Can you work these out from the model? Positions are in its coordinate system, mm. A direction names the side the tool comes from. Round coordinates to 2 decimals unless told otherwise and drop trailing zeros. Loops run counter-clockwise (first coordinate to the right, second up) from the corner with the lowest first, then second, coordinate; pieces in that order, holes last. Notation, with made-up numbers: (74, -2) -> (106, -2) arc R22 ccw to (106, 14) -> close; hole circle Ø7 at (-16.5, 78). An arc over 180 degrees is marked (long way). Answer as a JSON object with one key per item and string values.
```python
from build123d import *

# Parameters (mm, degrees)
SKETCH1_W           = 60
SKETCH1_H           = 45
BOSS_EXTRUDE1_DEPTH = 8
SKETCH2_R           = 5
CUT_EXTRUDE1_DEPTH  = 5
SKETCH3_W           = 20
SKETCH3_H           = 40
CUT_EXTRUDE2_DEPTH  = 5
SKETCH4_W           = 8
SKETCH4_H           = 45
BOSS_EXTRUDE3_DEPTH = 45
SKETCH6_R           = 1.5
CUT_EXTRUDE3_DEPTH  = 45
FILLET2_R           = 2
SKETCH7_R           = 14.99024042
CUT_EXTRUDE4_DEPTH  = 71.10884395


with BuildPart() as part:
    # Sketch1 → Boss-Extrude1 (new body)
    with BuildSketch(Plane(origin=(0, 0, 0), x_dir=(1, 0, 0), z_dir=(0, 1, 0))):
        Rectangle(SKETCH1_W, SKETCH1_H)
    extrude(amount=BOSS_EXTRUDE1_DEPTH)

    # Sketch2 → Cut-Extrude1 (cut)
    with BuildSketch(Plane.XZ):
        with Locations(Location((-20, 14.5, 0), (0, 0, 270))):
            Circle(SKETCH2_R)
        with Locations(Location((-20, -14.5, 0), (0, 0, 270))):
            Circle(SKETCH2_R)
    extrude(amount=-CUT_EXTRUDE1_DEPTH, mode=Mode.SUBTRACT)

    # Sketch3 → Cut-Extrude2 (cut)
    with BuildSketch(Plane.XZ):
        Rectangle(SKETCH3_W, SKETCH3_H)
    extrude(amount=-CUT_EXTRUDE2_DEPTH, mode=Mode.SUBTRACT)

    # Sketch4 → Boss-Extrude3 (add)
    with BuildSketch(Plane(origin=(0, 8, 0), x_dir=(1, 0, 0), z_dir=(0, 1, 0))):
        with Locations((-6, 0)):
            Rectangle(SKETCH4_W, SKETCH4_H)
    extrude(amount=BOSS_EXTRUDE3_DEPTH)

    # Sketch6 → Cut-Extrude3 (cut)
    with BuildSketch(Plane.ZY.offset(10)):
        with Locations((-15, 45.5)):
            Circle(SKETCH6_R)
        with Locations((15, 45.5)):
            Circle(SKETCH6_R)
        with Locations((15, 15.5)):
            Circle(SKETCH6_R)
        with Locations((-15, 15.5)):
            Circle(SKETCH6_R)
    extrude(amount=-CUT_EXTRUDE3_DEPTH, mode=Mode.SUBTRACT)

    # Fillet2
    fillet2_edges = [part.edges().sort_by_distance(p)[0] for p in [
        (-6, 53, -22.5),
        (-6, 53, 22.5),
    ]]
    fillet(fillet2_edges, radius=FILLET2_R)

    # Sketch7 → Cut-Extrude4 (cut, through all)
    with BuildSketch(Plane.ZY.offset(10)):
        with Locations((0, 30.5)):
            Circle(SKETCH7_R)
    extrude(amount=-CUT_EXTRUDE4_DEPTH, mode=Mode.SUBTRACT)


solid = part.part
```
Q1. We'd pull the mould along Z, two halves only. Please class faces 1 (the cylindrical face through (-24.88, 2.46, 15.58)), 2 (the flat face through (-2.4, 14, 22.5)), 3 (the flat face through (-6, 53, 0)): pulls with the +Z half, pulls with the -Z half, needs draft (parallel to the pull), parting line crosses it, or undercut.
Determined:
{"face 1": "undercut", "face 2": "pulls with the +Z half", "face 3": "needs draft"}
Q2. If I drill on L1, parallel to X at y = 2.5, z = 8.5; L2, parallel to X at y = 47, z = -10; L3, parallel to Y at x = -7, z = 0, over which ranges is the centre line in solid material (lowest first)? Write a range as [from, to].
Determined:
{"L1": "[-30, -10], [10, 30]", "L2": "[-10, -2]", "L3": "[5, 15.51], [45.49, 53]"}
Q3. I want a section at D-D, the plane z = 11. Write out the boundary of the cut face in (x, y).
Determined:
{"outline": "(-30, 0) -> (-23.57, 0) -> (-23.57, 5) -> (-16.43, 5) -> (-16.43, 0) -> (-10, 0) -> (-10, 5) -> (10, 5) -> (10, 0) -> (30, 0) -> (30, 8) -> (-2, 8) -> (-2, 20.32) -> (-10, 20.32) -> (-10, 8) -> (-30, 8) -> close; (-10, 40.68) -> (-2, 40.68) -> (-2, 53) -> (-10, 53) -> close"}
Q4. I want a section at C-C, the plane y = 33.5. Write out the boundary of the cut face in (x, z), then the cut area to 3 significant figures.
Determined:
{"outline": "(-10, -22.5) -> (-2, -22.5) -> (-2, -14.69) -> (-10, -14.69) -> close; (-10, 14.69) -> (-2, 14.69) -> (-2, 22.5) -> (-10, 22.5) -> close", "area": "125 mm²"}
Q5. I'm going to push flat-ended pins straight in: pin 1 (4 mm diameter, centred on y = 11.5, z = 7.5, fed in from +X); pin 2 (1.8 mm diameter, centred on y = 15.5, z = -15, fed in from -X); pin 3 (9 mm diameter, centred on x = -20, z = -14.5, fed in from +Y); pin 4 (10 mm diameter, centred on x = 1.5, z = 4.5, fed in from -Y). Where does each tip first touch, or does it pass through?
Determined:
{"pin 1": "x = -2", "pin 2": "through", "pin 3": "y = 8", "pin 4": "y = 5"}
Q6. On a 3-axis mill with a long thin cutter (end or side, diameter ignored), from which of +Z, -Z, +X, -X, +Y, -Y can I reach the whole of each face in a straight line? I mean faces 4 (the flat face through (-20, 8, 0)), 5 (the flat face through (14, 8, 0)), 6 (the flat face through (-20, 5, 15)), 7 (the cylindrical face through (-6.056, 45.363, -1.951)). Say none if no direction works.
Determined:
{"face 4": "+Z, -Z, -X, +Y", "face 5": "+Z, -Z, +X, +Y", "face 6": "-Y", "face 7": "+X, -X"}
Q7. I want a section at A-A, the plane x = 9. Write out the boundary of the cut face in (y, z), then the cut area to 3 significant figures.
Determined:
{"outline": "(0, -22.5) -> (8, -22.5) -> (8, 22.5) -> (0, 22.5) -> (0, 20) -> (5, 20) -> (5, -20) -> (0, -20) -> close", "area": "160 mm²"}
Q8. I want a section at B-B, the plane z = 4.5. Write out the boundary of the cut face in (x, y), then the cut area to 3 significant figures.
Determined:
{"outline": "(-30, 0) -> (-10, 0) -> (-10, 5) -> (10, 5) -> (10, 0) -> (30, 0) -> (30, 8) -> (-2, 8) -> (-2, 16.2) -> (-10, 16.2) -> (-10, 8) -> (-30, 8) -> close; (-10, 44.8) -> (-2, 44.8) -> (-2, 53) -> (-10, 53) -> close", "area": "511 mm²"}
